Check sheet for the modelled part. Datum: model origin and axes. Units: mm. Face numbers are marked on the shaded views. A direction names the side the tool comes from. Coordinates: 2 decimals unless noted, no trailing zeros. Write each loop counter-clockwise with the first axis right and the second up, starting at its lowest first coordinate (ties: lowest second). Pieces come first, ordered by that corner, then holes. Notation, with made-up numbers: (43.25, 0) -> (83.25, 0) arc R26 cw to (83.25, 24) -> close; hole circle Ø4 at (-14.75, 75.5). An arc over 180 degrees is marked (long way). Put each result on its own line as item: value.
```python
from build123d import *

# Parameters (mm, degrees)
SKETCH_1_W           = 135
SKETCH_1_H           = 80
EXTRUDE_1_DEPTH      = 70
SKETCH_6_W           = 45
SKETCH_6_H           = 70
CUT_EXTRUDE_1_DEPTH  = 35
SKETCH_5_W           = 45
SKETCH_5_H           = 70
CUT_EXTRUDE_2_DEPTH  = 35
SKETCH_7_W           = 80
SKETCH_7_H           = 70
CUT_EXTRUDE_3_DEPTH  = 75
SKETCH_8_W           = 87.8
SKETCH_8_H           = 77.8
SKETCH_8_W_2         = 82.2
SKETCH_8_H_2         = 72.2
CUT_EXTRUDE_4_DEPTH  = 10
SKETCH_9_R           = 5
CUT_EXTRUDE_5_DEPTH  = 32.4
SKETCH_10_W          = 21.5
SKETCH_10_H          = 15
CUT_EXTRUDE_6_DEPTH  = 10
SKETCH_12_W          = 16.99068276
SKETCH_12_H          = 10
CUT_EXTRUDE_7_DEPTH  = 45
CUT_EXTRUDE_8_DEPTH  = 3
SKETCH_15_W          = 10
SKETCH_15_H          = 10
CUT_EXTRUDE_9_DEPTH  = 6
SKETCH_17_R          = 1.095275866
CUT_EXTRUDE_11_DEPTH = 7
SKETCH_18_W          = 5
SKETCH_18_H          = 5
SKETCH_18_R          = 1.1
EXTRUDE_2_DEPTH      = 5
SKETCH_19_W          = 90
SKETCH_19_H          = 80
EXTRUDE_3_DEPTH      = 5


with BuildPart() as part:
    # 草圖1 → 填料-伸長1 (new body)
    with BuildSketch(Plane.XY):
        with Locations((-8.008902174, 5.58988764)):
            Rectangle(SKETCH_1_W, SKETCH_1_H)
    extrude(amount=EXTRUDE_1_DEPTH)

    # 草圖6 → 除料-伸長1 (cut)
    with BuildSketch(Plane(origin=(0, 45.58988764, 0), x_dir=(1, 0, 0), z_dir=(0, 1, 0))):
        with Locations((36.991097826, -35)):
            Rectangle(SKETCH_6_W, SKETCH_6_H)
    extrude(amount=-CUT_EXTRUDE_1_DEPTH, mode=Mode.SUBTRACT)

    # 草圖5 → 除料-伸長2 (cut)
    with BuildSketch(Plane.XZ.offset(34.41011236)):
        with Locations((36.991097826, 35)):
            Rectangle(SKETCH_5_W, SKETCH_5_H)
    extrude(amount=-CUT_EXTRUDE_2_DEPTH, mode=Mode.SUBTRACT)

    # 草圖7 → 除料-伸長3 (cut)
    with BuildSketch(Plane.XY):
        with Locations((-30.508902174, 5.58988764)):
            Rectangle(SKETCH_7_W, SKETCH_7_H)
    extrude(amount=CUT_EXTRUDE_3_DEPTH, mode=Mode.SUBTRACT)

    # 草圖8 → 除料-伸長4 (cut)
    with BuildSketch(Plane(origin=(0, 0, 0), x_dir=(-1, 0, 0), z_dir=(0, 0, -1))):
        with Locations((30.508902174, 5.58988764)):
            Rectangle(SKETCH_8_W, SKETCH_8_H)
        with Locations((30.508902174, 5.58988764)):
            Rectangle(SKETCH_8_W_2, SKETCH_8_H_2, mode=Mode.SUBTRACT)
    extrude(amount=-CUT_EXTRUDE_4_DEPTH, mode=Mode.SUBTRACT)

    # 草圖9 → 除料-伸長5 (cut)
    with BuildSketch(Plane(origin=(14.491097826, 0, 0), x_dir=(0, 0, -1), z_dir=(1, 0, 0))):
        with Locations((-55, 30.58988764)):
            Circle(SKETCH_9_R)
        with Locations((-20, -19.41011236)):
            Circle(SKETCH_9_R)
    extrude(amount=-CUT_EXTRUDE_5_DEPTH, mode=Mode.SUBTRACT)

    # 草圖10 → 除料-伸長6 (cut)
    with BuildSketch(Plane(origin=(0, -34.41011236, 0), x_dir=(-1, 0, 0), z_dir=(0, -1, 0))):
        with Locations((24.758902174, -18.5)):
            Rectangle(SKETCH_10_W, SKETCH_10_H)
    extrude(amount=-CUT_EXTRUDE_6_DEPTH, mode=Mode.SUBTRACT)

    # 草圖12 → 除料-伸長7 (cut)
    with BuildSketch(Plane(origin=(14.491097826, 0, 0), x_dir=(0, 0, -1), z_dir=(1, 0, 0))):
        with Locations((-61.50465862, 5.58988764)):
            Rectangle(SKETCH_12_W, SKETCH_12_H)
        with Locations((-8.49534138, 5.58988764)):
            Rectangle(SKETCH_12_W, SKETCH_12_H)
    extrude(amount=CUT_EXTRUDE_7_DEPTH, mode=Mode.SUBTRACT)

    # 草圖14 → 除料-伸長8 (cut)
    with BuildSketch(Plane(origin=(0, 0.58988764, 0), x_dir=(-1, 0, 0), z_dir=(0, -1, 0))):
        with BuildLine():
            Line((-38.009101008, -30.10282789), (-21.517914827, -33.5))
            ThreePointArc((-21.517914827, -33.5), (-20.017914827, -35), (-21.517914827, -36.5))
            Line((-21.517914827, -36.5), (-38.009101008, -39.89717211))
            ThreePointArc((-38.009101008, -39.89717211), (-39.017914827, -40), (-40.026728646, -39.89717211))
            Line((-40.026728646, -39.89717211), (-56.517914827, -36.5))
            ThreePointArc((-56.517914827, -36.5), (-58.017914827, -35), (-56.517914827, -33.5))
            Line((-56.517914827, -33.5), (-40.026728646, -30.10282789))
            ThreePointArc((-40.026728646, -30.10282789), (-39.017914827, -30), (-38.009101008, -30.10282789))
        make_face()
    extrude(amount=-CUT_EXTRUDE_8_DEPTH, mode=Mode.SUBTRACT)

    # 草圖15 → 除料-伸長9 (cut)
    with BuildSketch(Plane(origin=(0, 10.58988764, 0), x_dir=(1, 0, 0), z_dir=(0, 1, 0))):
        with Locations((39.491097826, -34.99068276)):
            Rectangle(SKETCH_15_W, SKETCH_15_H)
    extrude(amount=-CUT_EXTRUDE_9_DEPTH, mode=Mode.SUBTRACT)

    # 草圖17 → 除料-伸長11 (cut)
    with BuildSketch(Plane(origin=(0, 0.58988764, 0), x_dir=(-1, 0, 0), z_dir=(0, -1, 0))):
        with Locations((-39.017914827, -35)):
            Circle(SKETCH_17_R)
    extrude(amount=-CUT_EXTRUDE_11_DEPTH, mode=Mode.SUBTRACT)

    # 草圖18 → 填料-伸長2 (add)
    with BuildSketch(Plane.XY):
        with Locations((11.991097826, 48.08988764)):
            Rectangle(SKETCH_18_W, SKETCH_18_H)
        with Locations((11.991097826, 48.08988764)):
            Circle(SKETCH_18_R, mode=Mode.SUBTRACT)
        with Locations((-73.008902174, 48.08988764)):
            Rectangle(SKETCH_18_W, SKETCH_18_H)
        with Locations((-73.008902174, 48.08988764)):
            Circle(SKETCH_18_R, mode=Mode.SUBTRACT)
        with Locations((-73.008902174, -36.91011236)):
            Rectangle(SKETCH_18_W, SKETCH_18_H)
        with Locations((-73.008902174, -36.91011236)):
            Circle(SKETCH_18_R, mode=Mode.SUBTRACT)
        with Locations((11.991097826, -36.91011236)):
            Rectangle(SKETCH_18_W, SKETCH_18_H)
        with Locations((11.991097826, -36.91011236)):
            Circle(SKETCH_18_R, mode=Mode.SUBTRACT)
    extrude(amount=EXTRUDE_2_DEPTH)

    # 草圖19 → 填料-伸長3 (add)
    with BuildSketch(Plane.XY.offset(70)):
        with Locations((-30.508902174, 5.58988764)):
            Rectangle(SKETCH_19_W, SKETCH_19_H)
    extrude(amount=EXTRUDE_3_DEPTH)


solid = part.part
```
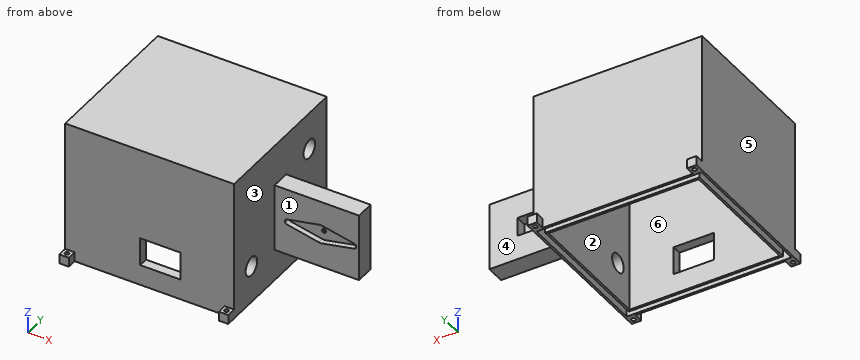
Q1. Cross-section at B-B (x = -27.5). Record the cut outline in (y, z), plus the area to 3 significant figures.
Recorded:
outline: (-34.41, 0) -> (-33.31, 0) -> (-33.31, 10) -> (-30.51, 10) -> (-30.51, 0) -> (-29.41, 0) -> (-29.41, 11) -> (-34.41, 11) -> close; (-34.41, 26) -> (-29.41, 26) -> (-29.41, 70) -> (40.59, 70) -> (40.59, 0) -> (41.69, 0) -> (41.69, 10) -> (44.49, 10) -> (44.49, 0) -> (45.59, 0) -> (45.59, 75) -> (-34.41, 75) -> close
area: 969 mm2
Q2. Depth check by flat-ended pin: P1, Ø3, axis at x = 39.5, y = 8, coming from the -Z side; P2, Ø8, axis at x = -9, z = 6, coming from the +Y side; P3, Ø1, axis at x = 4.5, z = 58.5, coming from the -Y side. Enter the tip coordinate at first touch or a pass-through.
Recorded:
P1: stops at z = 16.99
P2: stops at y = 45.59
P3: stops at y = -34.41
Q3. Material ranges on line 1 along X through (y, z) = (41, 9.5); line 2 along X through (y, z) = (-14, 19); line 3 along Y through (x, z) = (-9.5, 18), recorded low to high.
Recorded:
line 1: x = -75.51 to -74.41, -71.61 to 10.59, 13.39 to 14.49
line 2: x = -75.51 to -70.51, 9.49 to 14.49
line 3: y = -34.41 to -29.41, 40.59 to 45.59
Q4. Cross-section at A-A (z = 20). Record the cut outline in (x, y), plus the area to 3 significant figures.
Recorded:
outline: (-75.51, -34.41) -> (-35.51, -34.41) -> (-35.51, -29.41) -> (-70.51, -29.41) -> (-70.51, 40.59) -> (9.49, 40.59) -> (9.49, -14.41) -> (14.49, -14.41) -> (14.49, 0.59) -> (59.49, 0.59) -> (59.49, 10.59) -> (14.49, 10.59) -> (14.49, 45.59) -> (-75.51, 45.59) -> close; (-14.01, -34.41) -> (14.49, -34.41) -> (14.49, -24.41) -> (9.49, -24.41) -> (9.49, -29.41) -> (-14.01, -29.41) -> close
area: 1,890 mm2
Q5. Cross-section at D-D (y = 13). Record the cut outline in (x, z), plus the area to 3 significant figures.
Recorded:
outline: (-75.51, 0) -> (-74.41, 0) -> (-74.41, 10) -> (-71.61, 10) -> (-71.61, 0) -> (-70.51, 0) -> (-70.51, 70) -> (9.49, 70) -> (9.49, 0) -> (10.59, 0) -> (10.59, 10) -> (13.39, 10) -> (13.39, 0) -> (14.49, 0) -> (14.49, 75) -> (-75.51, 75) -> close
area: 1,090 mm2
Q6. Tool access check on the marked faces 4, 5 and 6. Record the directions out of +Z, -Z, +X, -X, +Y, -Y that give a thin tool (end or side, any length) a straight path to the whole face; none if there is none.
Recorded:
face 4: +Z, -Z, +X, +Y
face 5: +Z, -Z, -X, +Y, -Y
face 6: -Z
Q7. Cross-section at C-C (z = 47). Record the cut outline in (x, y), plus the area to 3 significant figures.
Recorded:
outline: (-75.51, -34.41) -> (14.49, -34.41) -> (14.49, 0.59) -> (59.49, 0.59) -> (59.49, 10.59) -> (14.49, 10.59) -> (14.49, 45.59) -> (-75.51, 45.59) -> close; hole (-70.51, -29.41) -> (9.49, -29.41) -> (9.49, 40.59) -> (-70.51, 40.59) -> close
area: 2,050 mm2
Q8. Mould release check, pull along Y, two halves, no side actions. Record for the marked faces 1, 2 and 3: released by +Y, released by -Y, zero draft, split by the parting line, or undercut.
Recorded:
face 1: released by -Y
face 2: undercut
face 3: zero draft
